Autodesk Inventor part; units mm, degrees
ref_plane "YZ Plane" through (0, 0, 0) normal (1, 0, 0) x (0, 1, 0)
ref_plane "XZ Plane" through (0, 0, 0) normal (0, 1, 0) x (-1, 0, 0)
ref_plane "XY Plane" through (0, 0, 0) normal (0, 0, 1) x (1, 0, 0)
sketch "Sketch1" plane through (0, 0, 0) normal (0, 1, 0) x (-1, 0, 0)
  circle A0 centre (0, 0) radius 12.5
  dimension "d0" = 25
extrude "Extrusion1" add sketch "Sketch1" along normal blind 53.7
hole "ReliefTop" at (0, 53.7, 0) direction (0, -1, 0) diameter 13.97 depth 0.254 countersink diameter 14.478 countersink angle 90
hole "ReliefBottom" at (0, 0, 0) direction (0, 1, 0) diameter 13.97 depth 0.254 countersink diameter 14.478 countersink angle 90
hole "MountBottomM6" at (0, 0.254, 0) direction (0, 1, 0) diameter 4.917 depth 7.366 tip angle 118 countersink diameter 5.508 countersink angle 90
hole "MountTopM4" at (0, 53.446, 0) direction (0, -1, 0) diameter 3.242 depth 14.478 tip angle 118 countersink diameter 3.808 countersink angle 90
sketch "Sketch2" plane through (0, 0, 0) normal (0, 0, 1) x (1, 0, 0)
  circle A0 centre (0, 20) radius 3
  line L0 (-12.5, 0) -> (12.5, 0)
  line L1 (0, -4.6) -> (0, 27.6)
  point P0 (0, 0)
  dimension "d49" = 6
  dimension "d50" = 20
extrude "Extrusion2" cut sketch "Sketch2" along normal through all both and the other way through all
chamfer "Chamfer1" distance 0.313 angle 45 2 edges at (-3, 19.9998, 12.1347) (-3, 19.9998, -12.1347)
equation "\"d1\" = height"
equation "\"d5\" = reliefMinor"
equation "\"d7\" = reliefMajor"
equation "\"d10\" = reliefDepth"
equation "\"d14\" = reliefMinor"
equation "\"d16\" = reliefMajor"
equation "\"d19\" = reliefDepth"
equation "\"d25\" = chamferM6"
equation "\"d28\" = depthM6"
equation "\"d40\" = chamferM4"
equation "\"d43\" = depthM4"
equation "\"reliefDepth\" = 0.254"
equation "\"reliefMinor\" = 13.97"
equation "\"reliefMajor\" = 14.478"
equation "\"chamferM6\" = 5.508"
equation "\"chamferM4\" = 3.808"
equation "\"depthM6\" = 7.366"
equation "\"depthM4\" = 14.478"
equation "\"height\" = 53.7"
properties part number "PLS-P642H0537A00_M" material "Stainless Steel"
Check sheet for the modelled part. Datum: model origin and axes. Units: mm. A direction names the side the tool comes from. Give positions to 0.01 mm unless a question says otherwise; leave off trailing zeros. Write each loop counter-clockwise with the first axis right and the second up, starting at its lowest first coordinate (ties: lowest second). Pieces come first, ordered by that corner, then holes. Notation, with made-up numbers: (48, 38) -> (72, 38) arc R36 cw to (72, 72) -> close; hole circle Ø3 at (77, -23). An arc over 180 degrees is marked (long way). Write item = value, one per line.
Item 1: Tool access check on faces 1 (the flat face through (1.5, 53.446, 1.5)), 2 (the flat face through (-5.4, 53.7, -5.4)), 3 (the cylindrical face through (-0.738, 4.134, -2.345)). Record the directions out of +Z, -Z, +X, -X, +Y, -Y that give a thin tool (end or side, any length) a straight path to the whole face; none if there is none.
Output:
face_1 = +Y
face_2 = +Z, -Z, +X, -X, +Y
face_3 = -Y
Item 2: Gauge pin test, flat ends, axial feed: pin 1 (4 mm diameter, centred on x = 3.5, z = 2, fed in from -Y); pin 2 (8 mm diameter, centred on y = 46.5, z = 8, fed in from -X); pin 3 (12 mm diameter, centred on x = -4, y = 8, fed in from +Z); pin 4 (1.5 mm diameter, centred on x = -3.5, z = -4, fed in from +Y). Record the tip position at first contact, or that the pin passes through.
Output:
pin_1 = 0.25
pin_2 = -11.84
pin_3 = 12.5
pin_4 = 53.45
Item 3: Scan lines: probe 1 along Z at (x, y) = (0, 43.5); probe 2 along Z at (x, y) = (0, 4); probe 3 along Y at (x, z) = (-0.25, -2.5). Record each from-to range of solid material in increasing order. Write a range as from..to.
Output:
probe_1 = -12.5..-1.62, 1.62..12.5
probe_2 = -12.5..-2.46, 2.46..12.5
probe_3 = 0.5..17.01, 22.99..53.45
Item 4: Sectioned sample at A-A on z = 10.25. Record the boundary of the cut face in (x, y), and give its area (3 significant figures).
Output:
outline = (-7.15, 0) -> (7.15, 0) -> (7.15, 53.7) -> (-7.15, 53.7) -> close; hole circle Ø6 at (0, 20)
area = 740 mm^2
Item 5: Release check for a two-part mould opening along Y. For faces 4 (the cylindrical face through (-0.65, 17.07, 0.17)), 5 (the conical face through (0.19, 38.163, -0.207)), 6 (the flat face through (0, 0.254, -3)) record: +Y half, -Y half, draft (parallel to the pull), parting line (faces both ways), or undercut.
Output:
face_4 = undercut
face_5 = +Y half
face_6 = -Y half
Item 6: Sectioned sample at B-B on y = 26.5. Record the boundary of the cut face in (x, z), and give its area (3 significant figures).
Output:
outline = circle Ø25 at (0, 0)
area = 491 mm^2
